Geometry check sheet. Reference: drawing and pictorial views, mm from the part's lowest x, y, z. A direction names the side the tool comes from. Give positions to 0.01 mm unless a question says otherwise; leave off trailing zeros. Order: outer loops, then holes, each group sorted by start corner. A loop starts at its lowest first (then second) coordinate and runs counter-clockwise, first axis right, second up. Notation, with made-up numbers: (69.5, 71.5) - (77.5, 71.5) arc R15 ccw to (77.5, 86.5) - close; hole circle Ø4 at (79, 11.5). An arc over 180 degrees is marked (long way). Answer in a Markdown table with one row per item.
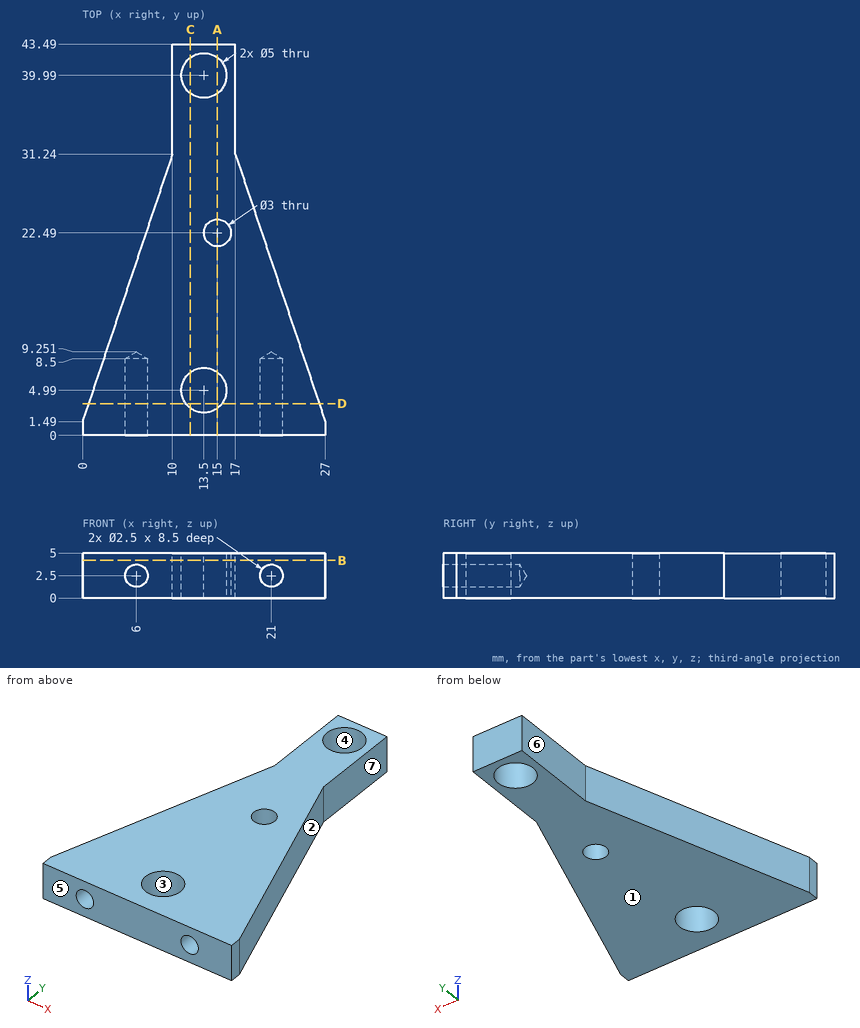
(1) Cross-section at B-B, the plane z = 4.2. Record the cut outline in (x, y).
Geometry says:
| item | result |
|---|---|
| outline | (0, 0) - (27, 0) - (27, 1.49) - (17, 31.24) - (17, 43.49) - (10, 43.49) - (10, 31.24) - (0, 1.49) - close; hole circle Ø5 at (13.5, 4.99); hole circle Ø5 at (13.5, 39.99); hole circle Ø3 at (15, 22.49) |
(2) Cross-section at D-D, the plane y = 3.5. Record the cut outline in (x, z).
Geometry says:
| item | result |
|---|---|
| outline | (0.68, 0) - (11.49, 0) - (11.49, 5) - (0.68, 5) - close; (15.51, 0) - (26.32, 0) - (26.32, 5) - (15.51, 5) - close; hole circle Ø2.5 at (6, 2.5); hole circle Ø2.5 at (21, 2.5) |
(3) Cross-section at A-A, the plane x = 15. Record the cut outline in (y, z), then the cut area to 3 significant figures.
Geometry says:
| item | result |
|---|---|
| outline | (0, 0) - (2.99, 0) - (2.99, 5) - (0, 5) - close; (6.99, 0) - (20.99, 0) - (20.99, 5) - (6.99, 5) - close; (23.99, 0) - (37.99, 0) - (37.99, 5) - (23.99, 5) - close; (41.99, 0) - (43.49, 0) - (43.49, 5) - (41.99, 5) - close |
| area | 162 mm² |
(4) Cross-section at C-C, the plane x = 12. Record the cut outline in (y, z).
Geometry says:
| item | result |
|---|---|
| outline | (0, 0) - (2.99, 0) - (2.99, 5) - (0, 5) - close; (6.99, 0) - (37.99, 0) - (37.99, 5) - (6.99, 5) - close; (41.99, 0) - (43.49, 0) - (43.49, 5) - (41.99, 5) - close |
(5) Thickness scan on L1, parallel to X at y = 6, z = 3.05; L2, parallel to X at y = 4.5, z = 3.25; L3, parallel to Y at x = 13, z = 3.4. Record the ranges inside material, lowest first.
Geometry says:
| item | result |
|---|---|
| L1 | 1.52 to 4.88, 7.12 to 11.21, 15.79 to 19.88, 22.12 to 25.48 |
| L2 | 1.01 to 5, 7 to 11.05, 15.95 to 20, 22 to 25.99 |
| L3 | 0 to 2.54, 7.44 to 37.54, 42.44 to 43.49 |
(6) Gauge pin test, flat end, axial feed: P1, Ø2.5, axis at y = 35.5, z = 2.5, coming from the -X side. Record the tip position at first contact, or that the pin passes through.
Geometry says:
| item | result |
|---|---|
| P1 | x = 10 |
(7) Mould release check, pull along X, two halves, no side actions. Record for the marked faces 1, 2, 3 and 4: pulls with the +X half, pulls with the -X half, needs draft (parallel to the pull), parting line crosses it, or undercut.
Geometry says:
| item | result |
|---|---|
| face 1 | needs draft |
| face 2 | pulls with the +X half |
| face 3 | undercut |
| face 4 | undercut |
(8) Access from +Z, -Z, +X, -X, +Y, -Y to the whole of each face (thin tool, end or side, straight path). Record for the marked faces 5, 6 and 7.
Geometry says:
| item | result |
|---|---|
| face 5 | +Z, -Z, +X, -X, -Y |
| face 6 | +Z, -Z, -X, +Y |
| face 7 | +Z, -Z, +X, +Y |
